Design review of the part built by this model. Coordinates are the model's own, in mm. Give positions to 0.01 mm unless a question says otherwise; leave off trailing zeros. Order: outer loops, then holes, each group sorted by start corner. A loop starts at its lowest first (then second) coordinate and runs counter-clockwise, first axis right, second up. Notation, with made-up numbers: (23, 53) -> (80, 53) arc R23 ccw to (80, 76) -> close; hole circle Ø2 at (-25.5, 46.25). An arc over 180 degrees is marked (long way). One line per item, written item: value.
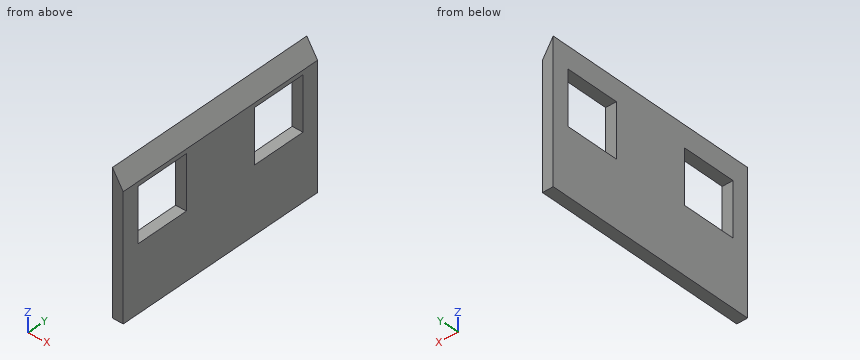
from build123d import *

# Parameters (mm, degrees)
F0_W        = 40
F0_H        = 26.199
F0_W_2      = 10
F0_H_2      = 10
F1_DEPTH    = 2
F2_T1_DEPTH = 56.5405413216


# Not quite as in the source:
# - a fillet or chamfer that OpenCascade refuses, or shapes differently, is made with other operations: its cross-section is extruded or revolved along the edge and cut away or added


with BuildPart() as f1:
    # F0 (on Right) → F1 (new body)
    with BuildSketch(Plane.YZ):
        Rectangle(F0_W, F0_H)
        with Locations((-12, 4.0995)):
            Rectangle(F0_W_2, F0_H_2, mode=Mode.SUBTRACT)
        with Locations((12, 4.0995)):
            Rectangle(F0_W_2, F0_H_2, mode=Mode.SUBTRACT)
    extrude(amount=F1_DEPTH)

    # F2: chamfer of 3.199 x 2.005940846 on 1 edges, made by hand

    # F2_s2 → F2_t1 (cut)
    with BuildSketch(Plane.XZ.offset(-28.2702706608)):
        Polygon((-0.005940846, 13.0995), (2, 9.9005), (2, 13.0995), align=None)
    extrude(amount=F2_T1_DEPTH, mode=Mode.SUBTRACT)


solid = f1.part
Item 1: To check wall thickness, follow line 1 along Y through (x, z) = (1.1, 4.5); line 2 along Z through (x, y) = (0.45, 7.5); line 3 along Z through (x, y) = (0.8, 11). State the ranges of each line that lie inside material, in increasing order. Write a range as from..to.
Returned:
line 1: -20..-17, -7..7, 17..20
line 2: -13.1..-0.9, 9.1..12.37
line 3: -13.1..-0.9, 9.1..11.81
Item 2: Add section D-D on y = -6. Give the boundary of the cut face in (x, z).
Returned:
outline: (0, -13.1) -> (2, -13.1) -> (2, 9.9) -> (0, 13.09) -> close
Item 3: Add section C-C on x = 1.3. Give the boundary of the cut face in (y, z).
Returned:
outline: (-20, -13.1) -> (20, -13.1) -> (20, 11.02) -> (-20, 11.02) -> close; hole (-17, -0.9) -> (-7, -0.9) -> (-7, 9.1) -> (-17, 9.1) -> close; hole (7, -0.9) -> (17, -0.9) -> (17, 9.1) -> (7, 9.1) -> close
Item 4: Add section A-A on y = -14.5. Give the boundary of the cut face in (x, z).
Returned:
outline: (0, -13.1) -> (2, -13.1) -> (2, -0.9) -> (0, -0.9) -> close; (0, 9.1) -> (2, 9.1) -> (2, 9.9) -> (0, 13.09) -> close
Item 5: Add section B-B on z = 7. Give the boundary of the cut face in (x, y), plus the area to 3 significant figures.
Returned:
outline: (0, -20) -> (2, -20) -> (2, -17) -> (0, -17) -> close; (0, -7) -> (2, -7) -> (2, 7) -> (0, 7) -> close; (0, 17) -> (2, 17) -> (2, 20) -> (0, 20) -> close
area: 40.0 mm²
Item 6: Clearance check with a flat-ended pin moving along its axis: P1, Ø1, axis at x = 1, y = -12, coming from the +Z side. State where the tip first meets the part, or that it passes through.
Returned:
P1: z = 12.29
